Autodesk Inventor part; units mm, degrees
ref_plane "YZ Plane" through (0, 0, 0) normal (1, 0, 0) x (0, 1, 0)
ref_plane "XZ Plane" through (0, 0, 0) normal (0, 1, 0) x (-1, 0, 0)
ref_plane "XY Plane" through (0, 0, 0) normal (0, 0, 1) x (1, 0, 0)
sketch "Sketch1" plane through (0, 0, 0) normal (0, 0, 1) x (1, 0, 0)
  circle A0 centre (0, 0) radius 96
  circle A1 centre (0, 0) radius 120
  dimension "d22" = 192
  dimension "d23" = 240
extrude "Plate1" add sketch "Sketch1" along normal blind 4
sketch "Sketch5" plane through (0, 0, 4) normal (0, 0, 1) x (1, 0, 0)
  circle A0 centre (0, 108) radius 5
  circle A1 centre (0, 0) radius 108 construction
  dimension "d25" = 216
  dimension "d24" = 10
extrude "Cut1" cut sketch "Sketch5" against normal blind 4
pattern_circular "Circular Pattern1" count 12 over 360 about axis through (0, 0, 0) along (0, 0, 1) of "Cut1"
equation "\"d26\" = Thickness"
equation "\"d2\" = Thickness"
equation "\"BendReliefWidth\" = Thickness"
equation "\"BendReliefDepth\" = 0.5 * Thickness"
equation "\"CornerReliefSize\" = 4 * Thickness"
equation "\"MinimumRemnant\" = 2 * Thickness"
equation "\"TransitionRadius\" = BendRadius"
equation "\"JacobiRadiusSize\" = BendRadius"
equation "\"GapSize\" = Thickness"
properties part number "TKS 3213 flange ffilter" material "Stainless Steel"
The listing builds one solid part. Answer for the finished solid, in the listing's coordinates (mm). Coordinates: 2 decimals unless noted, no trailing zeros. Loops run counter-clockwise (first coordinate to the right, second up) from the corner with the lowest first, then second, coordinate; pieces in that order, holes last. Notation, with made-up numbers: (88, 32.25) -> (119, 32.25) arc R8 ccw to (119, 37.25) -> close; hole circle Ø7 at (-24, 44.25). An arc over 180 degrees is marked (long way). Answer in a Markdown table with one row per item. Add a question column.
1. Flat-ended cylindrical pins translate along their axes: P1, Ø2, axis at y = -41, z = 0.5, coming from the +X side; P2, Ø2, axis at y = -29, z = 2.5, coming from the +X side; P3, Ø2, axis at y = 42, z = 0.5, coming from the +X side. Find the tip coordinate at first contact, or state that the pin passes through.
2. Determine the mould class of faces 1 (the flat face through (-1, -97, 0)), 2 (the cylindrical face through (1.08, -103.12, 2.03)), 3 (the cylindrical face through (-119.884, -5.276, 1.972)) for opening direction Y: +Y half, -Y half, draft (parallel to the pull), parting line (faces both ways), or undercut.
3. The part is cut by section D-D, the plane z = 1.1. Count the separate pieces of the cut face and the enclosed holes in it, then the cut area to 3 significant figures.
4. The part is cut by section C-C, the plane x = 69.5. Write down the section's boundary in (y, z) (3 decimals).
5. Consider line 1 (Y direction, x = 52, z = 2.5); line 2 (X direction, y = 6, z = 3.2); line 3 (X direction, y = -107, z = 3.1). Determine where each line is inside the solid, lowest interval first. Write a range as [from, to].
6. The part is cut by section B-B, the plane y = 42. Write down the section's boundary in (x, z), then the cut area to 3 significant figures.
7. The part is cut by section A-A, the plane x = 0. Write down the section's boundary in (y, z), then the cut area to 3 significant figures.
Answer below:
| question | item | result |
|---|---|---|
| 1 | P1 | x = 113.14 |
| 1 | P2 | x = 116.69 |
| 1 | P3 | x = 112.78 |
| 2 | face 1 | draft |
| 2 | face 2 | undercut |
| 2 | face 3 | parting line |
| 3 | separate pieces | 1 |
| 3 | enclosed holes | 13 |
| 3 | area | 15,300 mm2 |
| 4 | outline | (-97.825, 0) -> (-66.225, 0) -> (-66.225, 4) -> (-97.825, 4) -> close; (66.225, 0) -> (97.825, 0) -> (97.825, 4) -> (66.225, 4) -> close |
| 5 | line 1 | [-108.15, -98.11], [-88.95, -80.7], [80.7, 88.95], [98.11, 108.15] |
| 5 | line 2 | [-119.85, -95.81], [95.81, 119.85] |
| 5 | line 3 | [-54.32, -4.9], [4.9, 54.32] |
| 6 | outline | (-112.41, 0) -> (-86.32, 0) -> (-86.32, 4) -> (-112.41, 4) -> close; (86.32, 0) -> (112.41, 0) -> (112.41, 4) -> (86.32, 4) -> close |
| 6 | area | 209 mm2 |
| 7 | outline | (-120, 0) -> (-113, 0) -> (-113, 4) -> (-120, 4) -> close; (-103, 0) -> (-96, 0) -> (-96, 4) -> (-103, 4) -> close; (96, 0) -> (103, 0) -> (103, 4) -> (96, 4) -> close; (113, 0) -> (120, 0) -> (120, 4) -> (113, 4) -> close |
| 7 | area | 112 mm2 |
